Read the model definition and answer for the solid it produces. Units are mm, in the model's axes. Round coordinates to 2 decimals unless told otherwise and drop trailing zeros. Loops run counter-clockwise (first coordinate to the right, second up) from the corner with the lowest first, then second, coordinate; pieces in that order, holes last. Notation, with made-up numbers: M 38.25,-37 L 94.25,-37 A5 cw 94.25,-30 Z; hole C 16.5,69 d2. An arc over 180 degrees is marked long. Write each question's results on one line, items separated by ' | '.
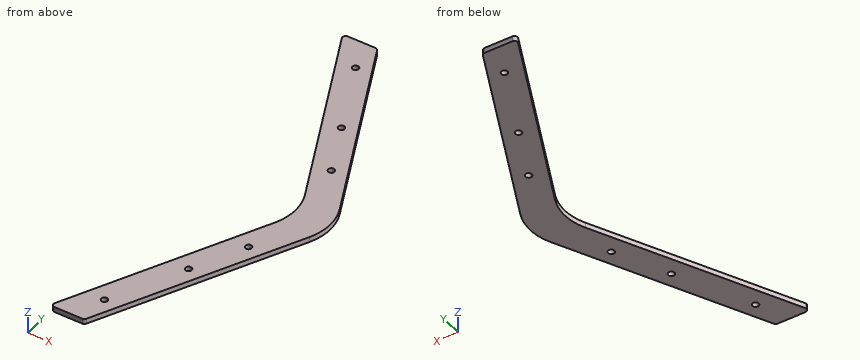
```python
from build123d import *

# Parameters (mm, degrees)
Y_KSEKLIK_EKSTR_ZYON1_DEPTH = 5
RADYUS1_R                   = 3
RADYUS2_R                   = 50
IZIM2_R                     = 3
KES_EKSTR_ZYON1_DEPTH       = 10


with BuildPart() as part:
    # Çizim1 → Yükseklik-Ekstrüzyon1 (new body)
    with BuildSketch(Plane.XY):
        Polygon((0, 209), (100, 0), (0, -209), (33.257168235, -209), (133.257168235, 0), (33.257168235, 209), align=None)
    extrude(amount=Y_KSEKLIK_EKSTR_ZYON1_DEPTH)

    # Radyus1
    radyus1_edges = [part.edges().sort_by_distance(p)[0] for p in [
        (0, -209, 2.5),
        (0, 209, 2.5),
        (33.257168235, 209, 2.5),
        (33.257168235, -209, 2.5),
    ]]
    fillet(radyus1_edges, radius=RADYUS1_R)

    # Radyus2
    radyus2_edges = [part.edges().sort_by_distance(p)[0] for p in [
        (100, 0, 2.5),
        (133.257168235, 0, 2.5),
    ]]
    fillet(radyus2_edges, radius=RADYUS2_R)

    # Çizim2 → Kes-Ekstrüzyon1 (cut)
    with BuildSketch(Plane.XY.offset(5)):
        with Locations((32.418057802, 179)):
            Circle(IZIM2_R)
        with Locations((65.910880768, 109)):
            Circle(IZIM2_R)
        with Locations((89.834325744, 59)):
            Circle(IZIM2_R)
        with Locations((89.834325744, -59)):
            Circle(IZIM2_R)
        with Locations((65.910880768, -109)):
            Circle(IZIM2_R)
        with Locations((32.418057802, -179)):
            Circle(IZIM2_R)
    extrude(amount=-KES_EKSTR_ZYON1_DEPTH, mode=Mode.SUBTRACT)


solid = part.part
```
1. Find the intervals of material crossed by L1, parallel to Y at x = 90.5, z = 2.4; L2, parallel to X at y = 179, z = 3.95; L3, parallel to Y at x = 49.5, z = 3.1 (3 decimals), in increasing order.
Completed:
L1: y = -89.36 to -61.93, -56.07 to -19.76, 19.76 to 56.07, 61.93 to 89.36 | L2: x = 14.35 to 29.42, 35.42 to 47.61 | L3: y = -175.052 to -105.545, 105.545 to 175.052
2. Find section D-D, the plane x = 117. Give the vertices of the cut face in (y, z).
Completed:
outline: M -33.98,0 L 33.98,0 L 33.98,5 L -33.98,5 Z
3. Find section B-B, the plane x = 54. Give the vertices of the cut face in (y, z).
Completed:
outline: M -165.65,0 L -96.14,0 L -96.14,5 L -165.65,5 Z; M 96.14,0 L 165.65,0 L 165.65,5 L 96.14,5 Z
4. Given P1, Ø5.5, axis at x = 89.83, y = -59, coming from the -Z side; P2, Ø1.5, axis at x = 44, z = 1.5, coming from the +Y side (3 decimals); P3, Ø3, axis at y = 49, z = 3.5, coming from the +X side; P4, Ø2, axis at x = 71.5, z = 1.5, coming from the +Y side, each flat-ended and moving along its own axis, determine where each tip first touches the part or whether it passes through.
Completed:
P1: passes through | P2: stops at y = 188.115 | P3: stops at x = 110.53 | P4: stops at y = 131.16
5. Find section A-A, the plane z = 2.3. Give the vertices of the cut face in (x, y), then the cut area to 3 significant figures.
Completed:
outline: M 2.05,-204.71 A3 ccw 4.76,-209 L 31.37,-209 A3 ccw 34.07,-207.29 L 122.93,-21.58 A50 ccw 122.93,21.58 L 34.07,207.29 A3 ccw 31.37,209 L 4.76,209 A3 ccw 2.05,204.71 L 89.67,21.58 A50 cw 89.67,-21.58 Z; hole C 32.42,-179 d6; hole C 32.42,179 d6; hole C 65.91,-109 d6; hole C 65.91,109 d6; hole C 89.83,-59 d6; hole C 89.83,59 d6 | area: 13,700 mm2
6. Find section C-C, the plane y = -82.5. Give the vertices of the cut face in (x, z), then the cut area to 3 significant figures.
Completed:
outline: M 60.53,0 L 93.78,0 L 93.78,5 L 60.53,5 Z | area: 166 mm2
